Design review of the part built by this model. Coordinates are the model's own, in mm. Face numbers are marked on the shaded views. A direction names the side the tool comes from. Coordinates: 2 decimals unless noted, no trailing zeros. Loops run counter-clockwise (first coordinate to the right, second up) from the corner with the lowest first, then second, coordinate; pieces in that order, holes last. Notation, with made-up numbers: (13.5, 82.5) - (45.5, 82.5) arc R24 cw to (45.5, 104.5) - close; hole circle Ø1 at (51, 30.25). An arc over 180 degrees is marked (long way). One line per question, with ' | ' between items.
from build123d import *

# Parameters (mm, degrees)
BOSS_EXTRUDE1_DEPTH       = 6.35
FILLET1_R                 = 2.54
F_6_CLEARANCE_HOLE1_D     = 3.6576
F_6_CLEARANCE_HOLE1_DEPTH = 10.16
F_6_CLEARANCE_HOLE1_TIP   = 1.0988539


with BuildPart() as part:
    # Sketch1 → Boss-Extrude1 (new body)
    with BuildSketch(Plane.XY):
        Polygon((0, 0), (7.296573321, 6.122551982), (31.02898218, -22.160631536), (31.02898218, -51.027448018), (21.50398218, -51.027448018), (21.50398218, -25.627448018), align=None)
    extrude(amount=BOSS_EXTRUDE1_DEPTH)

    # Fillet1
    fillet1_edges = [part.edges().sort_by_distance(p)[0] for p in [
        (0, 0, 3.175),
        (7.296573321, 6.122551982, 3.175),
        (31.02898218, -22.160631536, 3.175),
        (31.02898218, -51.027448018, 3.175),
        (21.50398218, -51.027448018, 3.175),
        (21.50398218, -25.627448018, 3.175),
    ]]
    fillet(fillet1_edges, radius=FILLET1_R)

    # #6 Clearance Hole1
    with Locations(Plane.XY.offset(6.35)):
        with Locations((7.729987982, -1.803106223), (26.26648218, -31.977448018)):
            Hole(F_6_CLEARANCE_HOLE1_D / 2, depth=F_6_CLEARANCE_HOLE1_DEPTH)
            with Locations((0, 0, -(F_6_CLEARANCE_HOLE1_DEPTH + F_6_CLEARANCE_HOLE1_TIP / 2))):  # 118° drill point
                Cone(0, F_6_CLEARANCE_HOLE1_D / 2, F_6_CLEARANCE_HOLE1_TIP, mode=Mode.SUBTRACT)


solid = part.part
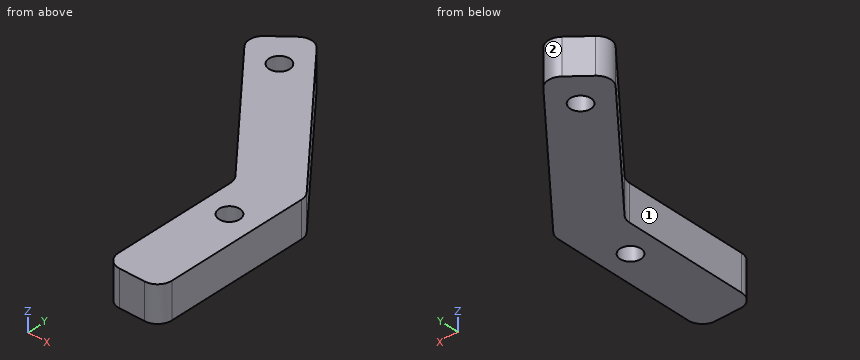
Q1. Tool access review of the marked faces 1 and 2: name each direction out of +Z, -Z, +X, -X, +Y, -Y from which nothing blocks a thin tool from reaching the whole face with its end or side.
Returned:
face 1: +Z, -Z, -X, -Y | face 2: +Z, -Z, +Y
Q2. For pin 1 (3 mm diameter, centred on x = 23, z = 2, fed in from +Y); pin 2 (3 mm diameter, centred on y = -32, z = 3, fed in from -X), all flat-tipped, find the tip position at first contact; note any pin that passes through.
Returned:
pin 1: stops at y = -10.8 | pin 2: stops at x = 21.5
Q3. Take a section at A-A (y = -33). Give the boundary of the cut face in (x, z), plus the area to 3 significant figures.
Returned:
outline: (21.5, 0) - (24.75, 0) - (24.75, 6.35) - (21.5, 6.35) - close; (27.78, 0) - (31.03, 0) - (31.03, 6.35) - (27.78, 6.35) - close | area: 41.2 mm²
Q4. Take a section at C-C (x = 25). Give the boundary of the cut face in (y, z), plus the area to 3 significant figures.
Returned:
outline: (-51.03, 0) - (-33.3, 0) - (-33.3, 6.35) - (-51.03, 6.35) - close; (-30.66, 0) - (-14.98, 0) - (-14.98, 6.35) - (-30.66, 6.35) - close | area: 212 mm²
Q5. Take a section at B-B (z = 1.75). Give the boundary of the cut face in (x, y).
Returned:
outline: (1.63, -1.95) - (20.91, -24.92) arc R2.54 cw to (21.5, -26.55) - (21.5, -48.49) arc R2.54 ccw to (24.04, -51.03) - (28.49, -51.03) arc R2.54 ccw to (31.03, -48.49) - (31.03, -23.09) arc R2.54 ccw to (30.43, -21.45) - (8.93, 4.18) arc R2.54 ccw to (5.35, 4.49) - (1.95, 1.63) arc R2.54 ccw to start; hole circle Ø3.66 at (7.73, -1.8); hole circle Ø3.66 at (26.27, -31.98)
Q6. To check wall thickness, follow line 1 along X through (y, z) = (-48, 0.75); line 2 along X through (y, z) = (-33, 3.5); line 3 along Y through (x, z) = (8, 4.5). State the ranges of each line that lie inside material, in increasing order.
Returned:
line 1: x = 21.5 to 31.03 | line 2: x = 21.5 to 24.75, 27.78 to 31.03 | line 3: y = -9.53 to -3.61, 0.01 to 4.87
Q7. Take a section at D-D (x = 17.5). Give the boundary of the cut face in (y, z), plus the area to 3 significant figures.
Returned:
outline: (-20.86, 0) - (-6.04, 0) - (-6.04, 6.35) - (-20.86, 6.35) - close | area: 94.1 mm²
